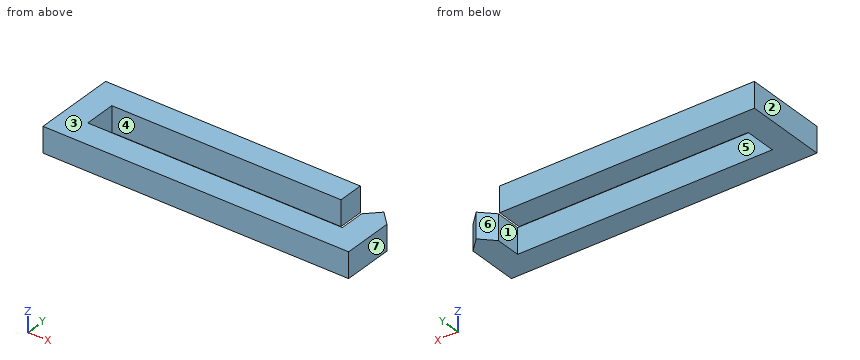
```python
from build123d import *

# Parameters (mm, degrees)
F0_W     = 4
F0_H     = 5
F0_H_2   = 5.9711672319
F1_DEPTH = 4
F2_SIZE  = 1.99999


# Not quite as in the source:
# - a fillet or chamfer is up to 0.001 mm smaller than in the source, because OpenCascade refuses the exact size


with BuildPart() as f1:
    # F0 (on Top) → F1 (new body)
    with BuildSketch(Plane.XY):
        with Locations((-21, -0.121395904)):
            Rectangle(F0_W, F0_H)
        Polygon((-19, -2.621395904), (-23, -2.621395904), (-23, -6.621395904), (25, -6.621395904), (25, -2.621395904), (21, -2.621395904), align=None)
        Polygon((-23, 6.378604096), (-23, 2.378604096), (-19, 2.378604096), (17, 2.378604096), (17, 6.378604096), align=None)
        with Locations((23, 0.364187712)):
            Rectangle(F0_W, F0_H_2)
    extrude(amount=F1_DEPTH)

    # F2 (size 2 in the source; OpenCascade refuses exactly that, so slightly less here)
    f2_edges = [f1.edges().sort_by_distance(p)[0] for p in [
        (21, 3.349771, 2),
        (25, 3.349771, 2),
    ]]
    chamfer(f2_edges, length=F2_SIZE)


solid = f1.part
```
Geometry: final body of the model. Coordinates: model frame, mm. Face numbers are marked on the shaded views. A direction names the side the tool comes from. Round coordinates to 2 decimals unless told otherwise and drop trailing zeros. Order: outer loops, then holes, each group sorted by start corner. A loop starts at its lowest first (then second) coordinate and runs counter-clockwise, first axis right, second up. Notation, with made-up numbers: (12.25, -7) - (26.25, -7) arc R34 cw to (26.25, 25) - close; hole circle Ø1 at (47.25, 77.5). An arc over 180 degrees is marked (long way). Write item = value, one per line. Start each with the question number.
Q1. Pull-direction query (X, two-part tool) for the marked faces 1, 2, 3 and 4; classes: +X half, -X half, draft (parallel to the pull), parting line (faces both ways), or undercut.
Q2. Ray query, line 1 (X direction, y = 0.25, z = 0.65); line 2 (Y direction, x = -17, z = 3.7); line 3 (X direction, y = 1.5, z = 2.15). Return the intervals inside material, ascending. Write a range as from..to.
Q3. Access query for the marked faces 5, 6 and 7. Directions: +Z, -Z, +X, -X, +Y, -Y. A direction counts if a zero-diameter tool reaches every point of the face in a straight line with its end or side. Return the directions, or none.
Q4. Cut plane B-B on y = -0.25. Return the cut outline in (x, z).
Q5. Cut plane A-A on x = -13. Return the cut outline in (y, z).
Outcome:
q1.face_1 = undercut
q1.face_2 = -X half
q1.face_3 = draft
q1.face_4 = undercut
q2.line_1 = -23..-19, 21..25
q2.line_2 = -6.62..-2.62, 2.38..6.38
q2.line_3 = -23..-19, 21.15..24.85
q3.face_5 = +Z, -Z
q3.face_6 = +Z, -Z, +Y
q3.face_7 = +Z, -Z, +X, +Y, -Y
q4.outline = (-23, 0) - (-19, 0) - (-19, 4) - (-23, 4) - close; (21, 0) - (25, 0) - (25, 4) - (21, 4) - close
q5.outline = (-6.62, 0) - (-2.62, 0) - (-2.62, 4) - (-6.62, 4) - close; (2.38, 0) - (6.38, 0) - (6.38, 4) - (2.38, 4) - close
